from build123d import *

# Parameters (mm, degrees)
BOSS_EXTRUDE1_DEPTH = 4.6
FILLET1_R           = 0.8


with BuildPart() as part:
    # BodySke → Base-Revolve (revolve)
    with BuildSketch(Plane.XY):
        with BuildLine():
            Line((3.0024, 8), (3.6, 8))
            Line((3.6, 8), (3.6, 3))
            Line((3.6, 3), (103.0455, 3))
            Line((103.0455, 3), (103.6, 2.4455))
            Line((103.6, 2.4455), (103.6, 0))
            Line((103.6, 0), (0, 0))
            ThreePointArc((0, 0), (0.775318389, 4.272423369), (3.0024, 8))
        make_face()
    revolve(axis=Axis((-31.75, 0, 0), (1, 0, 0)))

    # Sketch1 → Boss-Extrude1 (add)
    with BuildSketch(Plane(origin=(3.6, 0, 0), x_dir=(0, 0, -1), z_dir=(1, 0, 0))):
        Polygon((0, 4.242640687), (4.242640687, 0), (0, -4.242640687), (-4.242640687, 0), align=None)
    extrude(amount=BOSS_EXTRUDE1_DEPTH)

    # Sketch2 → Cut-Revolve1 (revolve, cut)
    with BuildSketch(Plane.XY):
        Polygon((8.2, 3), (13.2, 3), (13.2, 9), (2.2, 9), align=None)
    revolve(axis=Axis((0, 0, 0), (1, 0, 0)), mode=Mode.SUBTRACT)

    # Fillet1
    fillet1_edges = [part.edges().sort_by_distance(p)[0] for p in [
        (3.6, 2.121320344, -2.121320344),
        (3.6, -2.121320344, -2.121320344),
        (3.6, 2.121320344, 2.121320344),
        (3.6, -2.121320344, 2.121320344),
    ]]
    fillet(fillet1_edges, radius=FILLET1_R)


solid = part.part
For this review, take the finished solid that the model builds, in its own axes (mm). A direction names the side the tool comes from. Give positions to 0.01 mm unless a question says otherwise; leave off trailing zeros. Order: outer loops, then holes, each group sorted by start corner. A loop starts at its lowest first (then second) coordinate and runs counter-clockwise, first axis right, second up. Notation, with made-up numbers: (61, 70) - (115, 70) arc R18 ccw to (115, 97) - close; hole circle Ø2 at (80, 76.25). An arc over 180 degrees is marked (long way). Answer as a JSON object with one key per item and string values. Group by question number.
Item 1: Wall thickness on line 1 along Z through (x, y) = (14.5, 0); line 2 along X through (y, z) = (1.25, -6.75); line 3 along Y through (x, z) = (54, -1.5): over which ranges is each line inside the solid? List them lowest first.
Item 2: Take a section at A-A on x = 61.5. Give the boundary of the cut face in (y, z), and give its area (3 significant figures).
Item 3: Clearance check with flat-ended pins moving along their axes: pin 1 Ø6 at (y, z) = (3.5, -4) entering from -X; pin 2 Ø5 at (x, y) = (22, 4) entering from -Z; pin 3 Ø5 at (x, y) = (54.5, -0.5) entering from +Z; pin 4 Ø1 at (x, y) = (78.5, -4) entering from -Z. State where each tip first meets the part, or that it passes through.
Item 4: Machinability: for faces 1 (the flat face through (6.27, 2.09, 2.15)), 2 (the flat face through (6.27, -2.15, 2.09)), 3 (the flat face through (6.27, -2.09, -2.15)), which of the approach directions +Z, -Z, +X, -X, +Y, -Y give a long, thin tool a straight path to every point of the face, cutting with its end or side? Answer none if there is none.
Reported:
{
 "1": {"line 1": "-3 to 3", "line 2": "2.12 to 3.6", "line 3": "-2.6 to 2.6"},
 "2": {"outline": "circle Ø6 at (0, 0)", "area": "28.3 mm^2"},
 "3": {"pin 1": "x = 0.22", "pin 2": "z = -2.6", "pin 3": "z = 3", "pin 4": "through"},
 "4": {"face 1": "+Z, +X, +Y", "face 2": "+Z, +X, -Y", "face 3": "-Z, +X, -Y"}
}
